from build123d import *

# Parameters (mm, degrees)
SKETCH1_W           = 104.775
SKETCH1_H           = 71.12
SKETCH1_W_2         = 92.075
SKETCH1_H_2         = 58.42
BOSS_EXTRUDE1_DEPTH = 6.35
SKETCH1_3_W         = 104.775
SKETCH1_3_H         = 71.12
SKETCH1_3_W_2       = 92.075
SKETCH1_3_H_2       = 58.42
BOSS_EXTRUDE2_DEPTH = 38.1
CUT_EXTRUDE1_REACH  = 98.198
CUT_EXTRUDE2_REACH  = 119.021
SKETCH3_W           = 57.15
SKETCH3_H           = 22.86
BOSS_EXTRUDE3_DEPTH = 6.35
CUT_EXTRUDE3_REACH  = 79.984
SKETCH5_R           = 2.54
FILLET1_R           = 2.54


with BuildPart() as part:
    # Sketch1 → Boss-Extrude1 (new body)
    # profile 1 of 2: a face of its own
    with BuildSketch(Plane(origin=(0, 0, 0), x_dir=(1, 0, 0), z_dir=(0, 1, 0))):
        Rectangle(SKETCH1_W, SKETCH1_H)
        Rectangle(SKETCH1_W_2, SKETCH1_H_2, mode=Mode.SUBTRACT)
    # profile 2 of 2: a face of its own
    with BuildSketch(Plane(origin=(0, 0, 0), x_dir=(1, 0, 0), z_dir=(0, 1, 0))):
        Rectangle(SKETCH1_W_2, SKETCH1_H_2)
    extrude(amount=BOSS_EXTRUDE1_DEPTH)

    # Sketch1_3 → Boss-Extrude2 (add)
    with BuildSketch(Plane(origin=(0, 0, 0), x_dir=(1, 0, 0), z_dir=(0, 1, 0))):
        Rectangle(SKETCH1_3_W, SKETCH1_3_H)
        Rectangle(SKETCH1_3_W_2, SKETCH1_3_H_2, mode=Mode.SUBTRACT)
    extrude(amount=BOSS_EXTRUDE2_DEPTH)

    # Sketch2 → Cut-Extrude1 (cut, up to next)
    with BuildSketch(Plane.XY.offset(35.56), mode=Mode.PRIVATE) as cut_extrude1_sk1:
        with BuildLine():
            Line((-38.283663242, 19.05), (-2.723663242, 19.05))
            ThreePointArc((-2.723663242, 19.05), (3.626336758, 12.7), (-2.723663242, 6.35))
            Line((-2.723663242, 6.35), (-38.283663242, 6.35))
            ThreePointArc((-38.283663242, 6.35), (-44.633663242, 12.7), (-38.283663242, 19.05))
        make_face()
    cut_extrude1_tool1 = extrude(cut_extrude1_sk1.sketch, amount=-CUT_EXTRUDE1_REACH, mode=Mode.PRIVATE) & part.part
    add(cut_extrude1_tool1.solids().sort_by_distance((-20.503663, 12.7, 35.56))[0], mode=Mode.SUBTRACT)

    # Sketch3 → Cut-Extrude2 (cut, up to next)
    with BuildSketch(Plane(origin=(52.3875, 0, 0), x_dir=(0, 0, -1), z_dir=(1, 0, 0)), mode=Mode.PRIVATE) as cut_extrude2_sk1:
        with Locations((0.635, 17.78)):
            Rectangle(SKETCH3_W, SKETCH3_H)
    cut_extrude2_tool1 = extrude(cut_extrude2_sk1.sketch, amount=-CUT_EXTRUDE2_REACH, mode=Mode.PRIVATE) & part.part
    add(cut_extrude2_tool1.solids().sort_by_distance((52.3875, 17.78, -0.635))[0], mode=Mode.SUBTRACT)

    # Sketch4 → Boss-Extrude3 (add)
    with BuildSketch(Plane.XZ):
        with BuildLine():
            Line((-39.6875, 41.91), (-39.6875, 35.56))
            Line((-39.6875, 35.56), (-52.3875, 35.56))
            Line((-52.3875, 35.56), (-52.3875, 41.91))
            ThreePointArc((-52.3875, 41.91), (-46.0375, 48.26), (-39.6875, 41.91))
        make_face()
        with BuildLine():
            Line((39.6875, 41.91), (39.6875, 35.56))
            Line((39.6875, 35.56), (52.3875, 35.56))
            Line((52.3875, 35.56), (52.3875, 41.91))
            ThreePointArc((52.3875, 41.91), (46.0375, 48.26), (39.6875, 41.91))
        make_face()
        with BuildLine():
            Line((-52.3875, -41.91), (-52.3875, -35.56))
            Line((-52.3875, -35.56), (-39.6875, -35.56))
            Line((-39.6875, -35.56), (-39.6875, -41.91))
            ThreePointArc((-39.6875, -41.91), (-46.0375, -48.26), (-52.3875, -41.91))
        make_face()
        with BuildLine():
            Line((39.6875, -41.91), (39.6875, -35.56))
            Line((39.6875, -35.56), (52.3875, -35.56))
            Line((52.3875, -35.56), (52.3875, -41.91))
            ThreePointArc((52.3875, -41.91), (46.0375, -48.26), (39.6875, -41.91))
        make_face()
    extrude(amount=-BOSS_EXTRUDE3_DEPTH)

    # Sketch5 → Cut-Extrude3 (cut, up to next)
    with BuildSketch(Plane(origin=(0, 6.35, 0), x_dir=(1, 0, 0), z_dir=(0, 1, 0)), mode=Mode.PRIVATE) as cut_extrude3_sk1:
        with Locations(Location((-46.0375, 41.91, 0), (0, 0, 270))):
            Circle(SKETCH5_R)
    cut_extrude3_tool1 = extrude(cut_extrude3_sk1.sketch, amount=-CUT_EXTRUDE3_REACH, mode=Mode.PRIVATE) & part.part
    # Sketch5 → Cut-Extrude3 (cut, up to next)
    with BuildSketch(Plane(origin=(0, 6.35, 0), x_dir=(1, 0, 0), z_dir=(0, 1, 0)), mode=Mode.PRIVATE) as cut_extrude3_sk2:
        with Locations(Location((46.0375, 41.91, 0), (0, 0, 270))):
            Circle(SKETCH5_R)
    cut_extrude3_tool2 = extrude(cut_extrude3_sk2.sketch, amount=-CUT_EXTRUDE3_REACH, mode=Mode.PRIVATE) & part.part
    # Sketch5 → Cut-Extrude3 (cut, up to next)
    with BuildSketch(Plane(origin=(0, 6.35, 0), x_dir=(1, 0, 0), z_dir=(0, 1, 0)), mode=Mode.PRIVATE) as cut_extrude3_sk3:
        with Locations(Location((46.0375, -41.91, 0), (0, 0, 270))):
            Circle(SKETCH5_R)
    cut_extrude3_tool3 = extrude(cut_extrude3_sk3.sketch, amount=-CUT_EXTRUDE3_REACH, mode=Mode.PRIVATE) & part.part
    # Sketch5 → Cut-Extrude3 (cut, up to next)
    with BuildSketch(Plane(origin=(0, 6.35, 0), x_dir=(1, 0, 0), z_dir=(0, 1, 0)), mode=Mode.PRIVATE) as cut_extrude3_sk4:
        with Locations(Location((-46.0375, -41.91, 0), (0, 0, 270))):
            Circle(SKETCH5_R)
    cut_extrude3_tool4 = extrude(cut_extrude3_sk4.sketch, amount=-CUT_EXTRUDE3_REACH, mode=Mode.PRIVATE) & part.part
    add(cut_extrude3_tool1.solids().sort_by_distance((-46.0375, 6.35, -41.91))[0], mode=Mode.SUBTRACT)
    add(cut_extrude3_tool2.solids().sort_by_distance((46.0375, 6.35, -41.91))[0], mode=Mode.SUBTRACT)
    add(cut_extrude3_tool3.solids().sort_by_distance((46.0375, 6.35, 41.91))[0], mode=Mode.SUBTRACT)
    add(cut_extrude3_tool4.solids().sort_by_distance((-46.0375, 6.35, 41.91))[0], mode=Mode.SUBTRACT)

    # Fillet1
    fillet1_edges = [part.edges().sort_by_distance(p)[0] for p in [
        (-52.3875, 22.225, -35.56),
        (52.3875, 22.225, -35.56),
        (52.3875, 22.225, 35.56),
        (-52.3875, 22.225, 35.56),
    ]]
    fillet(fillet1_edges, radius=FILLET1_R)


solid = part.part
Can you work these out from the model? Positions are in its coordinate system, mm. A direction names the side the tool comes from. Round coordinates to 2 decimals unless told otherwise and drop trailing zeros. Order: outer loops, then holes, each group sorted by start corner. A loop starts at its lowest first (then second) coordinate and runs counter-clockwise, first axis right, second up. Notation, with made-up numbers: (-2.75, -0.75) - (48.25, -0.75) arc R27 ccw to (48.25, 27.25) - close; hole circle Ø11 at (70, 14). An arc over 180 degrees is marked (long way). Answer in a Markdown table with one row per item.
(1) Which directions (+Z, -Z, +X, -X, +Y, -Y) give clear straight access to the entire face, cutting with the end or side of a thin tool? Please do faces 4 (the face through (-21, 19.05, 32)), 5 (the face through (-51.62, 22.45, 34.84)), 6 (the face through (49, 18, 27.94)), 7 (the face through (46.038, 32, 2)), 8 (the face through (51.62, 22.45, 34.84)).
From the geometry:
| item | result |
|---|---|
| face 4 | +Z |
| face 5 | +Z, -X, +Y |
| face 6 | +X |
| face 7 | +Y |
| face 8 | +Z, +X, +Y |
(2) Please list where these lines run through material, in increasing order: L1, parallel to Z at x = -14, y = 24.5; L2, parallel to X at y = 4.25, z = -41.91; L3, parallel to X at y = 2, z = -41. Write a range as from..to.
From the geometry:
| item | result |
|---|---|
| L1 | z = -35.56..-29.21, 29.21..35.56 |
| L2 | x = -52.39..-48.58, -43.5..-39.69, 39.69..43.5, 48.58..52.39 |
| L3 | x = -52.39..-48.41, -43.67..-39.69, 39.69..43.67, 48.41..52.39 |
(3) Suppose I cut it at A-A, the plane y = 12.7. Please give me the cut outline in (x, z), plus the area to 3 significant figures.
From the geometry:
| item | result |
|---|---|
| outline | (-52.39, -33.02) arc R2.54 ccw to (-49.85, -35.56) - (49.85, -35.56) arc R2.54 ccw to (52.39, -33.02) - (52.39, -29.21) - (-46.04, -29.21) - (-46.04, 29.21) - (-44.63, 29.21) - (-44.63, 35.56) - (-49.85, 35.56) arc R2.54 ccw to (-52.39, 33.02) - close; (3.63, 29.21) - (46.04, 29.21) - (46.04, 27.94) - (52.39, 27.94) - (52.39, 33.02) arc R2.54 ccw to (49.85, 35.56) - (3.63, 35.56) - close |
| area | 1,400 mm2 |
(4) Suppose I cut it at C-C, the plane z = 7. Please give me the cut outline in (x, y).
From the geometry:
| item | result |
|---|---|
| outline | (-52.39, 0) - (52.39, 0) - (52.39, 6.35) - (-46.04, 6.35) - (-46.04, 38.1) - (-52.39, 38.1) - close; (46.04, 29.21) - (52.39, 29.21) - (52.39, 38.1) - (46.04, 38.1) - close |
(5) Suppose I cut it at B-B, the plane y = 5. Please give me the cut outline in (x, z), plus the area to 3 significant figures.
From the geometry:
| item | result |
|---|---|
| outline | (-52.39, -41.91) arc R6.35 ccw to (-39.69, -41.91) - (-39.69, -35.56) - (39.69, -35.56) - (39.69, -41.91) arc R6.35 ccw to (52.39, -41.91) - (52.39, 41.91) arc R6.35 ccw to (39.69, 41.91) - (39.69, 35.56) - (-39.69, 35.56) - (-39.69, 41.91) arc R6.35 ccw to (-52.39, 41.91) - close; hole circle Ø5.08 at (-46.04, -41.91); hole circle Ø5.08 at (-46.04, 41.91); hole circle Ø5.08 at (46.04, -41.91); hole circle Ø5.08 at (46.04, 41.91) |
| area | 7,950 mm2 |
(6) Suppose I cut it at D-D, the plane y = 31. Please give me the cut outline in (x, z), plus the area to 3 significant figures.
From the geometry:
| item | result |
|---|---|
| outline | (-52.39, -33.02) arc R2.54 ccw to (-49.85, -35.56) - (49.85, -35.56) arc R2.54 ccw to (52.39, -33.02) - (52.39, 33.02) arc R2.54 ccw to (49.85, 35.56) - (-49.85, 35.56) arc R2.54 ccw to (-52.39, 33.02) - close; hole (-46.04, -29.21) - (46.04, -29.21) - (46.04, 29.21) - (-46.04, 29.21) - close |
| area | 2,070 mm2 |
(7) If we mould it in two halves opening along Z, with no side actions, what happens to faces 1 (the face through (52.388, 6, 1)), 2 (the face through (-46.18, 3.13, 48.26)), 3 (the face through (-48.517, 3.219, -42.461))? For each: released by +Z, released by -Z, zero draft, split by the parting line, or undercut.
From the geometry:
| item | result |
|---|---|
| face 1 | zero draft |
| face 2 | released by +Z |
| face 3 | undercut |
(8) For P1, Ø5, axis at x = 15.5, y = 26, coming from the -Z side; P2, Ø9.5, axis at y = 21.5, z = 2, coming from the +X side; P3, Ø6.5, axis at x = 48, z = -41.5, coming from the +Y side, each with a flat end and sliding along its axis, tell me the tip position at first contact or that it passes through.
From the geometry:
| item | result |
|---|---|
| P1 | stops at z = -35.56 |
| P2 | stops at x = -46.04 |
| P3 | stops at y = 6.35 |
